from build123d import *

# Parameters (mm, degrees)
F0_W     = 76.464056
F0_H     = 115.89399
F0_R     = 35.376102
F1_DEPTH = 1000
F2_DEPTH = 600


with BuildPart() as f1:
    # F0 (on Front) → F1 (new body)
    with BuildSketch(Plane.XZ):
        Rectangle(F0_W, F0_H)
        with Locations((0.415236, -0.324309)):
            Circle(F0_R, mode=Mode.SUBTRACT)
        Polygon((38.232028, -125.84649), (38.232028, -57.946995), (-38.232028, -57.946995), (-38.232028, -124.745652), (-13.313413, -124.745652), (-13.313413, -103.494123), (14.12918, -104.132757), (14.12918, -124.888524), align=None)
    extrude(amount=F1_DEPTH)

    # F0 (on Front) → F2 (join)
    with BuildSketch(Plane.XZ):
        Rectangle(F0_W, F0_H)
        with Locations((0.415236, -0.324309)):
            Circle(F0_R, mode=Mode.SUBTRACT)
        Polygon((38.232028, -125.84649), (38.232028, -57.946995), (-38.232028, -57.946995), (-38.232028, -124.745652), (-13.313413, -124.745652), (-13.313413, -103.494123), (14.12918, -104.132757), (14.12918, -124.888524), align=None)
    extrude(amount=F2_DEPTH)


solid = f1.part
Read the model definition and answer for the solid it produces. Units are mm, in the model's axes. A direction names the side the tool comes from. Coordinates: 2 decimals unless noted, no trailing zeros. Order: outer loops, then holes, each group sorted by start corner. A loop starts at its lowest first (then second) coordinate and runs counter-clockwise, first axis right, second up. Notation, with made-up numbers: M 88,-6.5 L 117,-6.5 A10 cw 117,-0.5 Z; hole C -34.5,51 d7. An arc over 180 degrees is marked long. Put each result on its own line as item: value. Start each with the question number.
Item 1: Section A-A, the plane z = 10.5 is taken. Determine the outline of the cut face in (x, y), plus the area to 3 significant figures.
Item 2: Section C-C, the plane y = -361.5 is taken. Determine the outline of the cut face in (x, z), plus the area to 3 significant figures.
Item 3: The mould has two halves that part along X. Classify faces 1 (the face through (-1, -493, 57.947)), 2 (the face through (14.129, -493, -114)), 3 (the face through (-38.232, -493, -32)): +X half, -X half, draft (parallel to the pull), parting line (faces both ways), or undercut.
Item 4: Consider probe 1 along X at (y, z) = (-49, -3.5); probe 2 along X at (y, z) = (-810.5, -29); probe 3 along Z at (x, y) = (-28, -701.5). Determine where each line is inside the solid, lowest interval first. Write a range as [from, to].
Item 5: For faces 4 (the face through (-26, -493, -124.746)), 5 (the face through (-13.313, -493, -114)), 6 (the face through (38.232, -493, -35)), determine the directions among +Z, -Z, +X, -X, +Y, -Y from which every point of the face is accessible in a straight line to the end or side of a thin tool.
Item 6: Section B-B, the plane x = -25 is taken. Determine the outline of the cut face in (y, z).
Item 7: Given pin 1 Ø6 at (x, y) = (7.5, -369.5) entering from -Z; pin 2 Ø5 at (x, z) = (20, 23.5) entering from +Y; pin 3 Ø12.5 at (x, y) = (-25, -285) entering from -Z; pin 4 Ø1.5 at (x, y) = (12, -110.5) entering from -Z, each flat-ended and moving along its own axis, determine where each tip first touches the part or whether it passes through.
Computed:
1. outline: M -38.23,-1000 L -33.26,-1000 L -33.26,0 L -38.23,0 Z; M 34.09,-1000 L 38.23,-1000 L 38.23,0 L 34.09,0 Z
1. area: 9,110 mm2
2. outline: M -38.23,-124.75 L -13.31,-124.75 L -13.31,-103.49 L 14.13,-104.13 L 14.13,-124.89 L 38.23,-125.85 L 38.23,57.95 L -38.23,57.95 Z; hole C 0.42,-0.32 d70.75
2. area: 9,480 mm2
3. face 1: draft
3. face 2: undercut
3. face 3: -X half
4. probe 1: x = [-38.23, -34.82], [35.65, 38.23]
4. probe 2: x = [-38.23, -20.3], [21.13, 38.23]
4. probe 3: z = [-124.75, -21.4], [20.75, 57.95]
5. face 4: -Z, -X, +Y, -Y
5. face 5: -Z, +Y, -Y
5. face 6: +Z, -Z, +X, +Y, -Y
6. outline: M -1000,-124.75 L 0,-124.75 L 0,-24.93 L -1000,-24.93 Z; M -1000,24.28 L 0,24.28 L 0,57.95 L -1000,57.95 Z
7. pin 1: stops at z = -104.05
7. pin 2: passes through
7. pin 3: stops at z = -124.75
7. pin 4: stops at z = -104.1
